Can you work these out from the model? Positions are in its coordinate system, mm. A direction names the side the tool comes from. Give positions to 0.01 mm unless a question says otherwise; leave off trailing zeros. Order: outer loops, then holes, each group sorted by start corner. A loop starts at its lowest first (then second) coordinate and runs counter-clockwise, first axis right, second up. Notation, with made-up numbers: (33, 72) - (39, 72) arc R27 ccw to (39, 109) - close; hole circle Ø1 at (61.25, -35). An arc over 180 degrees is marked (long way). Return JSON: item names as keys, results as strings.
```python
from build123d import *

# Parameters (mm, degrees)
SKETCH_1_W                         = 7.5
SKETCH_1_H                         = 3.8
EXTRUDE_1_DEPTH                    = 6
CUT_EXTRUDE_1_DEPTH                = 5
CUT_EXTRUDE_2_DEPTH                = 11.329085148
EXTRUDE_2_REACH                    = 12.329
CUT_EXTRUDE_3_REACH                = 12.329
SKETCH_5_W                         = 5.3
SKETCH_5_H                         = 4.1
EXTRUDE_3_REACH                    = 11.972
EXTRUDE_5_REACH                    = 12.329
SKETCH_11_W                        = 2
SKETCH_11_H                        = 3.2
SKETCH_11_W_2                      = 0.8
SKETCH_11_H_2                      = 0.8
CUT_EXTRUDE_5_DEPTH                = 0.3
SKETCH_15_R                        = 0.05
CUT_EXTRUDE_6_DEPTH                = 0.1
CHAMFER_7_SIZE                     = 0.3
EXTRUDE_START                      = -4.8
SKETCH_7_W                         = 0.6
SKETCH_7_H                         = 0.6
EXTRUDE_4_DEPTH                    = 8
CHAMFER_6_SIZE                     = 0.2
PATTERN_LINEAR_1_COUNT             = 2
PATTERN_LINEAR_1_PITCH             = 2.5
CHAMFER_7_OF_PATTERN_LINEAR_1_SIZE = 0.3
CHAMFER_6_OF_PATTERN_LINEAR_1_SIZE = 0.2
CUT_EXTRUDE_4_REACH                = 11.972
CHAMFER_5_SIZE                     = 0.3


with BuildPart() as part:
    # Эскиз1 → Бобышка-Вытянуть1 (new body)
    with BuildSketch(Plane(origin=(0, 0, 0), x_dir=(1, 0, 0), z_dir=(0, 1, 0))):
        with Locations((3.75, -1.9)):
            Rectangle(SKETCH_1_W, SKETCH_1_H)
    extrude(amount=EXTRUDE_1_DEPTH)

    # Эскиз2 → Вырез-Вытянуть1 (cut)
    with BuildSketch(Plane(origin=(0, 6, 0), x_dir=(1, 0, 0), z_dir=(0, 1, 0))):
        Polygon((0.5, -0.5), (7, -0.5), (7, -1.5), (6.4, -1.5), (6.4, -3.3), (1.1, -3.3), (1.1, -1.5), (0.5, -1.5), align=None)
    extrude(amount=-CUT_EXTRUDE_1_DEPTH, mode=Mode.SUBTRACT)

    # Эскиз3 → Вырез-Вытянуть2 (cut, through all)
    with BuildSketch(Plane.ZY):
        Polygon((1.8, 6), (1.8, 1.5), (2.3, 1.5), (2.7, 3.459591794), (2.7, 3.821282026), (2.4, 4.085857157), (2.4, 4.385857157), (3.1, 5.1), (3.8, 5.1), (3.8, 6), align=None)
    extrude(amount=-CUT_EXTRUDE_2_DEPTH, mode=Mode.SUBTRACT)

    # Бобышка-Вытянуть2: up to this plane
    extrude_2_end = Plane(origin=(7.5, 5.1, 3.1), z_dir=(0, -0.6999999999999996, 0.7141428428542854))
    # Эскиз4 → Бобышка-Вытянуть2 (add, up to the surface)
    with BuildSketch(Plane.XY.offset(3.8), mode=Mode.PRIVATE) as extrude_2_sk1:
        with BuildLine():
            Line((0.3, 5.1), (0.8, 5.1))
            ThreePointArc((0.8, 5.1), (0.55, 5.35), (0.3, 5.1))
        make_face()
    extrude_2_tool1 = split(extrude(extrude_2_sk1.sketch, amount=-EXTRUDE_2_REACH, mode=Mode.PRIVATE), bisect_by=extrude_2_end, keep=Keep.BOTH, mode=Mode.PRIVATE)
    add(extrude_2_tool1.solids().sort_by_distance((0.55, 5.206103, 3.8))[0])

    # Эскиз5 → Вырез-Вытянуть3 (cut, up to next)
    with BuildSketch(Plane.XY.offset(3.8), mode=Mode.PRIVATE) as cut_extrude_3_sk1:
        with Locations((3.75, 3.05)):
            Rectangle(SKETCH_5_W, SKETCH_5_H)
    cut_extrude_3_tool1 = extrude(cut_extrude_3_sk1.sketch, amount=-CUT_EXTRUDE_3_REACH, mode=Mode.PRIVATE) & part.part
    add(cut_extrude_3_tool1.solids().sort_by_distance((3.75, 3.05, 3.8))[0], mode=Mode.SUBTRACT)

    # Эскиз6 → Бобышка-Вытянуть3 (add, up to next)
    with BuildSketch(Plane(origin=(0.5, 0, 0), x_dir=(0, 0, -1), z_dir=(1, 0, 0)), mode=Mode.PRIVATE) as extrude_3_sk1:
        Polygon((-2.9, 1), (-2.27, 1.5), (-0.5, 1.5), (-0.5, 1), align=None)
    extrude_3_tool1 = extrude(extrude_3_sk1.sketch, amount=EXTRUDE_3_REACH, mode=Mode.PRIVATE) - part.part
    add(extrude_3_tool1.solids().sort_by_distance((0.5, 1.23741, 1.550432))[0])

    # Эскиз9 → Бобышка-Вытянуть5 (add, up to next)
    with BuildSketch(Plane(origin=(0, 6, 0), x_dir=(1, 0, 0), z_dir=(0, 1, 0)), mode=Mode.PRIVATE) as extrude_5_sk1:
        Polygon((3.45, -0.5), (3.75, -0.928444402), (4.05, -0.5), align=None)
    extrude_5_tool1 = extrude(extrude_5_sk1.sketch, amount=-EXTRUDE_5_REACH, mode=Mode.PRIVATE) - part.part
    add(extrude_5_tool1.solids().sort_by_distance((3.75, 6, 0.642815))[0])

    # Эскиз11 → Вырез-Вытянуть5 (cut)
    with BuildSketch(Plane.XZ):
        with Locations((2.5, 1.6)):
            Rectangle(SKETCH_11_W, SKETCH_11_H)
        with Locations((2.5, 1.6)):
            Rectangle(SKETCH_11_W_2, SKETCH_11_H_2, mode=Mode.SUBTRACT)
    cut_extrude_5 = extrude(amount=-CUT_EXTRUDE_5_DEPTH, mode=Mode.SUBTRACT)

    # Эскиз15 → Вырез-Вытянуть6 (cut)
    with BuildSketch(Plane.XZ):
        with Locations(Location((2.5, 1.6, 0), (0, 0, 270))):
            Circle(SKETCH_15_R)
    extrude(amount=-CUT_EXTRUDE_6_DEPTH, mode=Mode.SUBTRACT)

    # Фаска7
    chamfer_7_edges = [part.edges().sort_by_distance(p)[0] for p in [
        (1.5, 0.3, 1.6),
        (2.5, 0.3, 3.2),
        (3.5, 0.3, 1.6),
        (2.9, 0.3, 1.6),
        (2.5, 0.3, 2),
        (2.1, 0.3, 1.6),
        (2.5, 0.3, 1.2),
    ]]
    chamfer(chamfer_7_edges, length=CHAMFER_7_SIZE - 0.0001)  # a hair under: the kernel refuses the full size

    # Эскиз7 → Бобышка-Вытянуть4 (add)
    with BuildSketch(Plane.XZ.offset(EXTRUDE_START)):
        with Locations((2.5, 1.6)):
            Rectangle(SKETCH_7_W, SKETCH_7_H)
    extrude_4 = extrude(amount=EXTRUDE_4_DEPTH)

    # Фаска6
    chamfer_6_edges = [part.edges().sort_by_distance(p)[0] for p in [
        (2.8, 4.8, 1.6),
        (2.5, 4.8, 1.9),
        (2.2, 4.8, 1.6),
        (2.5, 4.8, 1.3),
        (2.8, -3.2, 1.6),
        (2.5, -3.2, 1.9),
        (2.2, -3.2, 1.6),
        (2.5, -3.2, 1.3),
    ]]
    chamfer(chamfer_6_edges, length=CHAMFER_6_SIZE)

    # Линейный массив1: Вырез-Вытянуть5, Бобышка-Вытянуть4 ×2
    with Locations(*[(i * PATTERN_LINEAR_1_PITCH, 0, 0) for i in range(1, PATTERN_LINEAR_1_COUNT)]):
        add(cut_extrude_5, mode=Mode.SUBTRACT)
        add(extrude_4)

    # Фаска7 of Линейный массив1
    chamfer_7_of_pattern_linear_1_edges = [part.edges().sort_by_distance(p)[0] for p in [
        (4, 0.3, 1.6),
        (5, 0.3, 3.2),
        (6, 0.3, 1.6),
        (5.4, 0.3, 1.6),
        (5, 0.3, 2),
        (4.6, 0.3, 1.6),
        (5, 0.3, 1.2),
    ]]
    chamfer(chamfer_7_of_pattern_linear_1_edges, length=CHAMFER_7_OF_PATTERN_LINEAR_1_SIZE - 0.0001)  # a hair under: the kernel refuses the full size

    # Фаска6 of Линейный массив1
    chamfer_6_of_pattern_linear_1_edges = [part.edges().sort_by_distance(p)[0] for p in [
        (5.3, 4.8, 1.6),
        (5, 4.8, 1.9),
        (4.7, 4.8, 1.6),
        (5, 4.8, 1.3),
        (5.3, -3.2, 1.6),
        (5, -3.2, 1.9),
        (4.7, -3.2, 1.6),
        (5, -3.2, 1.3),
    ]]
    chamfer(chamfer_6_of_pattern_linear_1_edges, length=CHAMFER_6_OF_PATTERN_LINEAR_1_SIZE)

    # Вырез-Вытянуть4: up to this face of the body (flat: up to its plane)
    cut_extrude_4_end = Plane(part.part.faces().sort_by_distance((7, 3.75, 1))[0])
    # Эскиз10 → Вырез-Вытянуть4 (cut, up to the picked face)
    with BuildSketch(Plane(origin=(0.5, 0, 0), x_dir=(0, 0, -1), z_dir=(1, 0, 0)), mode=Mode.PRIVATE) as cut_extrude_4_sk1:
        Polygon((-1, 6), (-0.2, 6), (-1, 5.2), (-1, 5.1), (-1.8, 5.1), (-1.8, 6), align=None)
    cut_extrude_4_tool1 = split(extrude(cut_extrude_4_sk1.sketch, amount=CUT_EXTRUDE_4_REACH, mode=Mode.PRIVATE), bisect_by=cut_extrude_4_end, keep=Keep.BOTH, mode=Mode.PRIVATE)
    add(cut_extrude_4_tool1.solids().sort_by(Axis((0.5, 5.60641, 1.194872), (1, 0, 0)))[0], mode=Mode.SUBTRACT)

    # Фаска5
    chamfer_5_edges = [part.edges().sort_by_distance(p)[0] for p in [
        (7, 6, 1),
        (0.5, 6, 1),
    ]]
    chamfer(chamfer_5_edges, length=CHAMFER_5_SIZE)


solid = part.part
```
1. Suppose I cut it at B-B (x = 1.25). List the corners of the cut face in (y, z) for me.
Checks:
{"outline": "(0, 0) - (6, 0) - (6, 0.2) - (5.7, 0.5) - (1.5, 0.5) - (1.5, 2.27) - (1, 2.9) - (1, 3.8) - (0, 3.8) - close"}
2. Thinking about a two-plate mould opening in X: for faces 1 (the face through (1.1, 3, 3)), 2 (the face through (0.5, 3.3, 1.8)), 3 (the face through (7.5, 3, 1.5)), which applies, +X half, -X half, draft (parallel to the pull), parting line (faces both ways), or undercut?
Checks:
{"face 1": "undercut", "face 2": "draft", "face 3": "+X half"}
3. On a 3-axis mill with a long thin cutter (end or side, diameter ignored), from which of +Z, -Z, +X, -X, +Y, -Y can I reach the whole of each face in a straight line? I mean faces 4 (the face through (0.54, 2.47, 2.5)), 5 (the face through (2, 4, 0.5)), 6 (the face through (6.4, 3, 3)). Say none if no direction works.
Checks:
{"face 4": "+X, -X", "face 5": "+Y", "face 6": "+Z, +Y"}
4. For pin 1 Ø1 at (x, y) = (3.5, 4) entering from +Z; pin 2 Ø0.9 at (x, y) = (5.5, 4) entering from +Z; pin 3 Ø0.6 at (x, z) = (7, 3.5) entering from +Y, each with a flat end and sliding along its axis, tell me the tip position at first contact or that it passes through.
Checks:
{"pin 1": "z = 0.93", "pin 2": "z = 1.9", "pin 3": "y = 5.1"}
5. Suppose I cut it at C-C (y = 4.5). State how many separate pieces and enclosed holes the cut face has, plus the area to 3 significant figures.
Checks:
{"separate pieces": "5", "enclosed holes": "0", "area": "9.09 mm^2"}
6. If I drill on L1, parallel to X at y = 2, z = 2.6; L2, parallel to Z at x = 4.75, y = 3.5; L3, parallel to X at y = 1.75, z = 1.15, over which ranges is the centre line in solid material (lowest first)? Write a range as [from, to].
Checks:
{"L1": "[0, 1.1], [6.4, 7.5]", "L2": "[0, 0.5], [1.3, 1.9]", "L3": "[0, 0.5], [7, 7.5]"}
7. Suppose I cut it at D-D (x = 6.5). List the corners of the cut face in (y, z) for me, plus the area to 3 significant figures.
Checks:
{"outline": "(0, 0) - (6, 0) - (6, 0.2) - (5.7, 0.5) - (1.5, 0.5) - (1.5, 1.5) - (5.1, 1.5) - (5.1, 1.8) - (1.5, 1.8) - (1.5, 2.3) - (3.46, 2.7) - (3.82, 2.7) - (4.09, 2.4) - (4.39, 2.4) - (5.1, 3.1) - (5.1, 3.8) - (0, 3.8) - close", "area": "13.4 mm^2"}
8. Suppose I cut it at A-A (y = -1). List the corners of the cut face in (x, z) for me, plus the area to 3 significant figures.
Checks:
{"outline": "(2.2, 1.3) - (2.8, 1.3) - (2.8, 1.9) - (2.2, 1.9) - close; (4.7, 1.3) - (5.3, 1.3) - (5.3, 1.9) - (4.7, 1.9) - close", "area": "0.720 mm^2"}
